The listing builds one solid part. Answer for the finished solid, in the listing's coordinates (mm). Face numbers are marked on the shaded views. A direction names the side the tool comes from. Give positions to 0.01 mm unless a question says otherwise; leave off trailing zeros. Order: outer loops, then holes, each group sorted by start corner. A loop starts at its lowest first (then second) coordinate and runs counter-clockwise, first axis right, second up. Notation, with made-up numbers: M 18.5,51.5 L 71.5,51.5 A18 cw 71.5,59.5 Z; hole C 46,-33 d2. An arc over 180 degrees is marked long. Answer as a JSON object with one key per item and string values. Group by question number.
```python
from build123d import *

# Parameters (mm, degrees)
SKETCH1_W           = 40
SKETCH1_H           = 20
SKETCH1_R           = 1.6
BOSS_EXTRUDE1_DEPTH = 5
BOSS_EXTRUDE2_DEPTH = 2.5
BOSS_EXTRUDE3_DEPTH = 20
CUT_EXTRUDE1_DEPTH  = 2.5
CUT_EXTRUDE2_DEPTH  = 20
FILLET1_R           = 4
CHAMFER1_SIZE       = 1


with BuildPart() as part:
    # Sketch1 → Boss-Extrude1 (new body)
    with BuildSketch(Plane.XY):
        with Locations((20, 10)):
            Rectangle(SKETCH1_W, SKETCH1_H)
        with Locations((13, 10)):
            Circle(SKETCH1_R, mode=Mode.SUBTRACT)
        with Locations((34, 10)):
            Circle(SKETCH1_R, mode=Mode.SUBTRACT)
    extrude(amount=BOSS_EXTRUDE1_DEPTH)

    # Sketch3 → Boss-Extrude2 (add)
    with BuildSketch(Plane.XY.offset(5)):
        Polygon((35.58771324, 7.25), (36.38156986, 8.625), (37.175426481, 10), (36.38156986, 11.375), (35.58771324, 12.75), (0, 12.75), (0, 20), (40, 20), (40, 0), (0, 0), (0, 7.25), align=None)
    extrude(amount=BOSS_EXTRUDE2_DEPTH)

    # Sketch4 → Boss-Extrude3 (add, through all)
    with BuildSketch(Plane(origin=(0, 20, 0), x_dir=(1, 0, 0), z_dir=(0, 1, 0))):
        Polygon((40, -7.5), (0, -25), (0, -7.5), align=None)
    extrude(amount=-BOSS_EXTRUDE3_DEPTH)

    # Sketch6 → Cut-Extrude1 (cut)
    with BuildSketch(Plane.ZY):
        with BuildLine():
            Line((0, 10), (0, 6))
            Line((0, 6), (14, 6))
            ThreePointArc((14, 6), (18, 10), (14, 14))
            Line((14, 14), (0, 14))
            Line((0, 14), (0, 10))
        make_face()
    extrude(amount=-CUT_EXTRUDE1_DEPTH, mode=Mode.SUBTRACT)

    # Sketch7 → Cut-Extrude2 (cut)
    with BuildSketch(Plane(origin=(0, 0, 0), x_dir=(-1, 0, 0), z_dir=(0, 0, -1))):
        Polygon((-2.5, 14), (-2.5, 16), (-9.5, 16), (-9.5, 4), (-2.5, 4), (-2.5, 6), align=None)
    extrude(amount=-CUT_EXTRUDE2_DEPTH, mode=Mode.SUBTRACT)

    # Fillet1
    fillet1_edges = [part.edges().sort_by_distance(p)[0] for p in [
        (40, 10, 7.5),
        (20, 0, 16.25),
        (20, 20, 16.25),
        (40, 20, 3.75),
        (40, 0, 3.75),
    ]]
    fillet(fillet1_edges, radius=FILLET1_R)

    # Chamfer1
    chamfer1_edges = [part.edges().sort_by_distance(p)[0] for p in [
        (2.5, 14, 7),
        (2.5, 10, 18),
        (2.5, 6, 7),
        (9.5, 12.75, 6.25),
        (9.5, 7.25, 6.25),
        (2.5, 5, 0),
        (2.5, 15, 0),
        (6, 4, 0),
        (9.5, 10, 5),
        (9.5, 10, 7.5),
        (9.5, 10, 0),
        (6, 16, 0),
    ]]
    chamfer(chamfer1_edges, length=CHAMFER1_SIZE)


solid = part.part
```
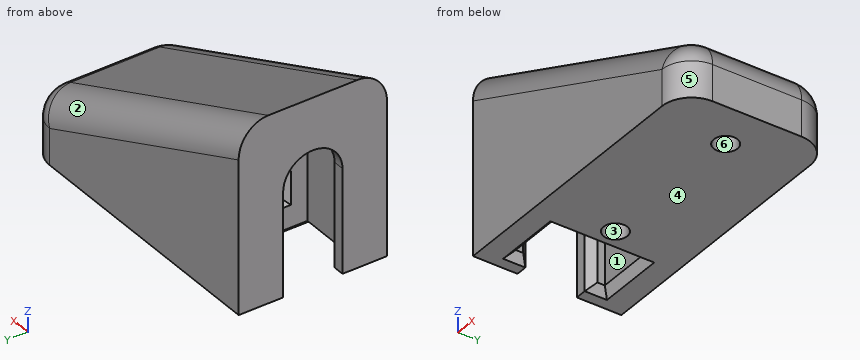
Item 1: Determine the mould class of the marked faces 1, 2, 3 and 4 for opening direction X: released by +X, released by -X, zero draft, split by the parting line, or undercut.
Item 2: Consider probe 1 along Y at (x, z) = (7, 12.5); probe 2 along Y at (x, z) = (13, 1.3); probe 3 along Z at (x, y) = (22, 12) (3 decimals). Determine where each line is inside the solid, lowest interval first. Write a range as from..to.
Item 3: A tool of negligible diameter and unlimited length cuts with its end or side. For the marked faces 5 and 6, from which of +Z, -Z, +X, -X, +Y, -Y can it reach the whole face along a straight path? Write none if from no direction.
Item 4: Flat-ended cylindrical pins translate along their axes: P1, Ø5, axis at y = 10, z = 8, coming from the -X side; P2, Ø4.5, axis at x = 29, y = 11, coming from the -Z side; P3, Ø1, axis at x = 35, z = 11.5, coming from the -Y side; P4, Ø2, axis at x = 4.5, y = 9.5, coming from the -Z side. Find the tip coordinate at first contact, or state that the pin passes through.
Item 5: Section A-A (z = 3.5) is taken. Determine the outline of the cut face in (x, y), and give its area (3 significant figures).
Values found:
{
 "1": {"face 1": "undercut", "face 2": "released by +X", "face 3": "undercut", "face 4": "zero draft"},
 "2": {"probe 1": "y = 0..4, 16..20", "probe 2": "y = 0..8.4, 11.6..20", "probe 3": "z = 0..5, 7.5..15.375"},
 "3": {"face 5": "+Z, -Z, +X, -Y", "face 6": "-Z"},
 "4": {"P1": "stops at x = 9.5", "P2": "stops at z = 0", "P3": "passes through", "P4": "stops at z = 20"},
 "5": {"outline": "M 0,0 L 36,0 A4 ccw 40,4 L 40,16 A4 ccw 36,20 L 0,20 L 0,14 L 1.5,14 L 2.5,15 L 2.5,16 L 9.5,16 L 9.5,4 L 2.5,4 L 2.5,5 L 1.5,6 L 0,6 Z; hole C 13,10 d3.2; hole C 34,10 d3.2", "area": "672 mm^2"}
}
